from build123d import *

# Parameters (mm, degrees)
SKETCH_W     = 48
SKETCH_H     = 28
PAD_DEPTH    = 2
SKETCH001_R  = 1
PAD001_DEPTH = 3
SKETCH002_W  = 21
SKETCH002_H  = 1
PAD002_DEPTH = 2


with BuildPart() as part:
    # Sketch → Pad (new body)
    with BuildSketch(Plane.XY):
        with Locations((24, 14)):
            Rectangle(SKETCH_W, SKETCH_H)
    extrude(amount=PAD_DEPTH)

    # Sketch001 → Pad001 (new body)
    with BuildSketch(Plane.XY.offset(2)):
        with Locations((2.2, 2.2)):
            Circle(SKETCH001_R)
        with Locations((2.2, 25.8)):
            Circle(SKETCH001_R)
        with Locations((45.8, 25.8)):
            Circle(SKETCH001_R)
        with Locations((45.8, 2.2)):
            Circle(SKETCH001_R)
    extrude(amount=PAD001_DEPTH)

    # Sketch002 → Pad002 (new body)
    with BuildSketch(Plane.XY.offset(2)):
        with Locations((20.5, 22.5)):
            Rectangle(SKETCH002_W, SKETCH002_H)
        with Locations((20.5, 5.5)):
            Rectangle(SKETCH002_W, SKETCH002_H)
    extrude(amount=PAD002_DEPTH)


solid = part.part
For this review, take the finished solid that the model builds, in its own axes (mm). A direction names the side the tool comes from. Give positions to 0.01 mm unless a question says otherwise; leave off trailing zeros. Loops run counter-clockwise (first coordinate to the right, second up) from the corner with the lowest first, then second, coordinate; pieces in that order, holes last. Notation, with made-up numbers: M 16,-38 L 33,-38 A27 ccw 33,-21 Z; hole C 53.25,-21.75 d8. An arc over 180 degrees is marked long. Answer as a JSON object with one key per item and string values. Group by question number.
Q1. For probe 1 along Y at (x, z) = (25.5, 2.95); probe 2 along Z at (x, y) = (9, 10.75); probe 3 along X at (y, z) = (25, 3.55), list the stretches that pass through material, from the lowest coordinate up. Write a range as [from, to].
Q2. Add section D-D on y = 24.25. Give the boundary of the cut face in (x, z), and give its area (3 significant figures).
Q3. Add section C-C on x = 2.2. Give the boundary of the cut face in (y, z), and give its area (3 significant figures).
Q4. Insertion check: P1, Ø1.1, axis at y = 22.5, z = 3, coming from the +X side; P2, Ø1.1, axis at y = 22.5, z = 3, coming from the -X side; P3, Ø1.6, axis at x = 23.5, z = 3.5, coming from the -Y side. Each pin has a flat end and moves straight along its axis. Give the tip position at first contact, or say it passes through.
Q5. Add section B-B on y = 2.2. Give the boundary of the cut face in (x, z), and give its area (3 significant figures).
Q6. Mouldability with a two-part tool opening along Y and no side actions: class faces 1 (the flat face through (24, 0, 1)), 2 (the flat face through (24, 28, 1)), 3 (the cylindrical face through (1.983, 24.824, 3.479)), 4 (the flat face through (31, 22.5, 3)) as +Y half, -Y half, draft (parallel to the pull), parting line (faces both ways), or undercut.
Q7. Tool access review of faces 5 (the flat face through (46, 2, 5)), 6 (the cylindrical face through (2.07, 3.19, 3.48)), 7 (the flat face through (20, 6, 3)), 8 (the flat face through (31, 5.5, 3)), 9 (the flat face through (10, 5.5, 3)): name each direction out of +Z, -Z, +X, -X, +Y, -Y from which nothing blocks a thin tool from reaching the whole face with its end or side.
Q8. Add section A-A on z = 3.35. Give the boundary of the cut face in (x, y), and give its area (3 significant figures).
Checked values:
{
 "1": {"probe 1": "[5, 6], [22, 23]", "probe 2": "[0, 2]", "probe 3": "[1.6, 2.8], [45.2, 46.4]"},
 "2": {"outline": "M 0,0 L 48,0 L 48,2 L 0,2 Z", "area": "96.0 mm²"},
 "3": {"outline": "M 0,0 L 28,0 L 28,2 L 26.8,2 L 26.8,5 L 24.8,5 L 24.8,2 L 3.2,2 L 3.2,5 L 1.2,5 L 1.2,2 L 0,2 Z", "area": "68.0 mm²"},
 "4": {"P1": "x = 31", "P2": "x = 10", "P3": "y = 5"},
 "5": {"outline": "M 0,0 L 48,0 L 48,2 L 46.8,2 L 46.8,5 L 44.8,5 L 44.8,2 L 3.2,2 L 3.2,5 L 1.2,5 L 1.2,2 L 0,2 Z", "area": "108 mm²"},
 "6": {"face 1": "-Y half", "face 2": "+Y half", "face 3": "undercut", "face 4": "draft"},
 "7": {"face 5": "+Z, +X, -X, +Y, -Y", "face 6": "+Z", "face 7": "+Z, +X, -X", "face 8": "+Z, +X, +Y, -Y", "face 9": "+Z, -X, +Y, -Y"},
 "8": {"outline": "C 2.2,2.2 d2; C 2.2,25.8 d2; M 10,5 L 31,5 L 31,6 L 10,6 Z; M 10,22 L 31,22 L 31,23 L 10,23 Z; C 45.8,2.2 d2; C 45.8,25.8 d2", "area": "54.6 mm²"}
}
